The model under review builds one solid part; all positions refer to its coordinate system, in mm. Round coordinates to 2 decimals unless told otherwise and drop trailing zeros. Loops run counter-clockwise (first coordinate to the right, second up) from the corner with the lowest first, then second, coordinate; pieces in that order, holes last. Notation, with made-up numbers: (89.5, 19) -> (118.5, 19) arc R8 ccw to (118.5, 33) -> close; hole circle Ø1 at (-11.75, -1). An arc over 180 degrees is marked (long way). Use a Markdown table: item, result. Add a question column.
1) Insertion check: pin 1 (1.5 mm diameter, centred on y = 2, z = 0.5, fed in from -X); pin 2 (3.5 mm diameter, centred on x = -185, z = -188, fed in from -Y). Each pin has a flat end and moves straight along its axis. Give the tip position at first contact, or say it passes through.
2) Consider section A-A on z = 0. Give the boundary of the cut face in (x, y), plus the area to 3 significant figures.
3) Wall thickness on probe 1 along Z at (x, y) = (185, 1.65); probe 2 along X at (y, z) = (2.3, 0); probe 3 along X at (y, z) = (2.2, 188): over which ranges is each line inside the solid? List them lowest first.
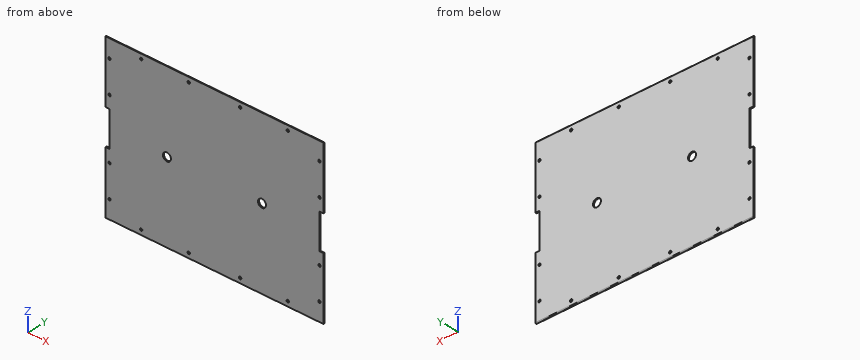
from build123d import *

# Parameters (mm, degrees)
SKETCH_1_R      = 3
SKETCH_1_R_2    = 10
EXTRUDE_1_DEPTH = 3
FILLET_1_R      = 2
FILLET_2_R      = 2


with BuildPart() as part:
    # 草图1 → 凸台-拉伸1 (new body)
    with BuildSketch(Plane(origin=(0, 0, 0), x_dir=(1, 0, 0), z_dir=(0, 1, 0))):
        Polygon((-275, -200), (275, -200), (275, -44), (265.5, -44), (265.5, 44), (275, 44), (275, 200), (-275, 200), (-275, 44), (-265.5, 44), (-265.5, -44), (-275, -44), align=None)
        with Locations(Location((-265, -75, 0), (0, 0, 270))):
            Circle(SKETCH_1_R, mode=Mode.SUBTRACT)
        with Locations(Location((-265, -155, 0), (0, 0, 270))):
            Circle(SKETCH_1_R, mode=Mode.SUBTRACT)
        with Locations(Location((-185, -188, 0), (0, 0, 270))):
            Circle(SKETCH_1_R, mode=Mode.SUBTRACT)
        with Locations(Location((-65, -188, 0), (0, 0, 270))):
            Circle(SKETCH_1_R, mode=Mode.SUBTRACT)
        with Locations(Location((-65, 188, 0), (0, 0, 270))):
            Circle(SKETCH_1_R, mode=Mode.SUBTRACT)
        with Locations(Location((-185, 188, 0), (0, 0, 270))):
            Circle(SKETCH_1_R, mode=Mode.SUBTRACT)
        with Locations(Location((-265, 155, 0), (0, 0, 270))):
            Circle(SKETCH_1_R, mode=Mode.SUBTRACT)
        with Locations(Location((-265, 75, 0), (0, 0, 270))):
            Circle(SKETCH_1_R, mode=Mode.SUBTRACT)
        with Locations(Location((265, 75, 0), (0, 0, 270))):
            Circle(SKETCH_1_R, mode=Mode.SUBTRACT)
        with Locations(Location((265, 155, 0), (0, 0, 270))):
            Circle(SKETCH_1_R, mode=Mode.SUBTRACT)
        with Locations(Location((185, 188, 0), (0, 0, 270))):
            Circle(SKETCH_1_R, mode=Mode.SUBTRACT)
        with Locations(Location((65, 188, 0), (0, 0, 270))):
            Circle(SKETCH_1_R, mode=Mode.SUBTRACT)
        with Locations(Location((65, -188, 0), (0, 0, 270))):
            Circle(SKETCH_1_R, mode=Mode.SUBTRACT)
        with Locations(Location((185, -188, 0), (0, 0, 270))):
            Circle(SKETCH_1_R, mode=Mode.SUBTRACT)
        with Locations(Location((265, -155, 0), (0, 0, 270))):
            Circle(SKETCH_1_R, mode=Mode.SUBTRACT)
        with Locations(Location((265, -75, 0), (0, 0, 270))):
            Circle(SKETCH_1_R, mode=Mode.SUBTRACT)
        with Locations(Location((-120, 0, 0), (0, 0, 270))):
            Circle(SKETCH_1_R_2, mode=Mode.SUBTRACT)
        with Locations(Location((120, 0, 0), (0, 0, 270))):
            Circle(SKETCH_1_R_2, mode=Mode.SUBTRACT)
    extrude(amount=EXTRUDE_1_DEPTH)

    # 圆角1
    fillet_1_edges = [part.edges().sort_by_distance(p)[0] for p in [
        (0, 3, 200),
    ]]
    fillet(fillet_1_edges, radius=FILLET_1_R)

    # 圆角2
    fillet_2_edges = [part.edges().sort_by_distance(p)[0] for p in [
        (0, 3, -200),
    ]]
    fillet(fillet_2_edges, radius=FILLET_2_R)


solid = part.part
Result set:
| question | item | result |
|---|---|---|
| 1 | pin 1 | x = -265.5 |
| 1 | pin 2 | through |
| 2 | outline | (-265.5, 0) -> (-130, 0) -> (-130, 3) -> (-265.5, 3) -> close; (-110, 0) -> (110, 0) -> (110, 3) -> (-110, 3) -> close; (130, 0) -> (265.5, 0) -> (265.5, 3) -> (130, 3) -> close |
| 2 | area | 1,470 mm2 |
| 3 | probe 1 | -199.89 to -191, -185 to 185, 191 to 199.89 |
| 3 | probe 2 | -265.5 to -130, -110 to 110, 130 to 265.5 |
| 3 | probe 3 | -275 to -188, -182 to -68, -62 to 62, 68 to 182, 188 to 275 |
